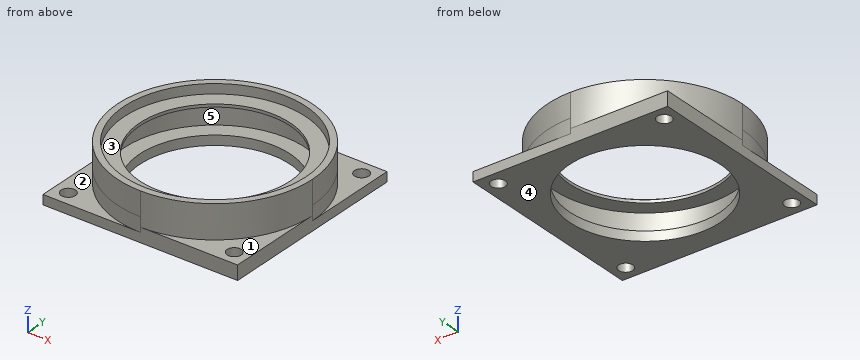
from build123d import *

# Parameters (mm, degrees)
SKETCH2_R               = 20.4
SKETCH2_R_2             = 15.75
SKETCH2_R_3             = 1.5
BOSS_EXTRUDE1_DEPTH     = 5
BOSS_EXTRUDE2_START     = 5
SKETCH2_4_R             = 20.4
SKETCH2_4_R_2           = 15.75
SKETCH2_4_R_3           = 1.5
BOSS_EXTRUDE2_DEPTH     = 6
SKETCH4_R               = 19.05
CUT_EXTRUDE2_DEPTH      = 3
CUT_EXTRUDE3_START      = -6
SKETCH5_R               = 19.05
SKETCH5_R_2             = 15.75
CUT_EXTRUDE3_DEPTH      = 5.4
CUT_EXTRUDE4_START      = -3
CUT_EXTRUDE4_DEPTH      = 3
CUT_EXTRUDE5_START      = -1
SKETCH7_R               = 19.05
CUT_EXTRUDE5_DEPTH      = 1
CUT_EXTRUDE6_DEPTH      = 30.938603842
CUT_EXTRUDE6_DEPTH_BACK = 5


with BuildPart() as part:
    # Sketch2 → Boss-Extrude1 (new body)
    # profile 1 of 5: a face of its own
    with BuildSketch(Plane.XY):
        Circle(SKETCH2_R)
        Circle(SKETCH2_R_2, mode=Mode.SUBTRACT)
    # profile 2 of 5: a face of its own
    with BuildSketch(Plane.XY):
        with BuildLine():
            Line((-20.4, 20.4), (-20.4, -3.8e-08))
            ThreePointArc((-20.4, -3.8e-08), (-14.424978339, 14.424978334), (3.1e-08, 20.4))
            Line((3.1e-08, 20.4), (-20.4, 20.4))
        make_face()
        with Locations((-17.4, 17.4)):
            Circle(SKETCH2_R_3, mode=Mode.SUBTRACT)
    # profile 3 of 5: a face of its own
    with BuildSketch(Plane.XY):
        with BuildLine():
            ThreePointArc((3.1e-08, 20.4), (14.424978347, 14.424978325), (20.4, 0))
            Line((20.4, 0), (20.4, 20.4))
            Line((20.4, 20.4), (3.1e-08, 20.4))
        make_face()
        with Locations((17.4, 17.4)):
            Circle(SKETCH2_R_3, mode=Mode.SUBTRACT)
    # profile 4 of 5: a face of its own
    with BuildSketch(Plane.XY):
        with BuildLine():
            ThreePointArc((20.4, 0), (14.424978335, -14.424978337), (-2e-09, -20.4))
            Line((-2e-09, -20.4), (20.4, -20.4))
            Line((20.4, -20.4), (20.4, 0))
        make_face()
        with Locations((17.4, -17.4)):
            Circle(SKETCH2_R_3, mode=Mode.SUBTRACT)
    # profile 5 of 5: a face of its own
    with BuildSketch(Plane.XY):
        with BuildLine():
            Line((-20.4, -3.8e-08), (-20.4, -20.4))
            Line((-20.4, -20.4), (-2e-09, -20.4))
            ThreePointArc((-2e-09, -20.4), (-14.424978323, -14.424978349), (-20.4, -3.8e-08))
        make_face()
        with Locations((-17.4, -17.4)):
            Circle(SKETCH2_R_3, mode=Mode.SUBTRACT)
    extrude(amount=BOSS_EXTRUDE1_DEPTH)

    # Sketch2<4> → Boss-Extrude2 (add)
    # profile 1 of 3: a face of its own
    with BuildSketch(Plane.XY.offset(BOSS_EXTRUDE2_START)):
        Circle(SKETCH2_4_R)
        Circle(SKETCH2_4_R_2, mode=Mode.SUBTRACT)
    # profile 2 of 3: a face of its own
    with BuildSketch(Plane.XY.offset(BOSS_EXTRUDE2_START)):
        with BuildLine():
            Line((-20.4, 20.4), (-20.4, -3.8e-08))
            ThreePointArc((-20.4, -3.8e-08), (-14.424978339, 14.424978334), (3.1e-08, 20.4))
            Line((3.1e-08, 20.4), (-20.4, 20.4))
        make_face()
        with Locations((-17.4, 17.4)):
            Circle(SKETCH2_4_R_3, mode=Mode.SUBTRACT)
    # profile 3 of 3: a face of its own
    with BuildSketch(Plane.XY.offset(BOSS_EXTRUDE2_START)):
        with BuildLine():
            ThreePointArc((20.4, 0), (14.424978335, -14.424978337), (-2e-09, -20.4))
            Line((-2e-09, -20.4), (20.4, -20.4))
            Line((20.4, -20.4), (20.4, 0))
        make_face()
        with Locations((17.4, -17.4)):
            Circle(SKETCH2_4_R_3, mode=Mode.SUBTRACT)
    extrude(amount=BOSS_EXTRUDE2_DEPTH)

    # Sketch4 → Cut-Extrude2 (cut)
    with BuildSketch(Plane.XY.offset(11)):
        Circle(SKETCH4_R)
    extrude(amount=-CUT_EXTRUDE2_DEPTH, mode=Mode.SUBTRACT)

    # Sketch5 → Cut-Extrude3 (cut)
    with BuildSketch(Plane.XY.offset(8).offset(CUT_EXTRUDE3_START)):
        Circle(SKETCH5_R)
        with Locations(Location((0, 0, 0), (0, 0, 180))):
            Circle(SKETCH5_R_2, mode=Mode.SUBTRACT)
    extrude(amount=CUT_EXTRUDE3_DEPTH, mode=Mode.SUBTRACT)

    # Sketch6 → Cut-Extrude4 (cut)
    with BuildSketch(Plane.XY.offset(5).offset(CUT_EXTRUDE4_START)):
        with BuildLine():
            Line((20.4, 0), (20.4, 20.4))
            Line((20.4, 20.4), (0, 20.4))
            ThreePointArc((0, 20.4), (14.424978336, 14.424978336), (20.4, 0))
        make_face()
        with BuildLine():
            Line((-20.4, 0), (-20.4, -20.4))
            Line((-20.4, -20.4), (0, -20.4))
            ThreePointArc((0, -20.4), (-14.424978336, -14.424978336), (-20.4, 0))
        make_face()
    extrude(amount=CUT_EXTRUDE4_DEPTH, mode=Mode.SUBTRACT)

    # Sketch7 → Cut-Extrude5 (cut)
    with BuildSketch(Plane.XY.offset(11).offset(CUT_EXTRUDE5_START)):
        with BuildLine():
            Line((20.4, -20.4), (20.4, 0))
            ThreePointArc((20.4, 0), (14.424978336, 14.424978336), (0, 20.4))
            Line((0, 20.4), (-20.4, 20.4))
            Line((-20.4, 20.4), (-20.4, 0))
            ThreePointArc((-20.4, 0), (-14.424978336, -14.424978336), (0, -20.4))
            Line((0, -20.4), (20.4, -20.4))
        make_face()
        Circle(SKETCH7_R, mode=Mode.SUBTRACT)
    extrude(amount=CUT_EXTRUDE5_DEPTH, mode=Mode.SUBTRACT)

    # Sketch8 → Cut-Extrude6 (cut, two sides: drawn at the far end of the back side and taken through both)
    with BuildSketch(Plane.XY.offset(8).offset(-CUT_EXTRUDE6_DEPTH_BACK)):
        with BuildLine():
            Line((-20.4, 20.4), (-20.4, 0))
            ThreePointArc((-20.4, 0), (-14.424978336, 14.424978336), (0, 20.4))
            Line((0, 20.4), (-20.4, 20.4))
        make_face()
        with BuildLine():
            ThreePointArc((20.4, 0), (14.424978336, -14.424978336), (0, -20.4))
            Line((0, -20.4), (20.4, -20.4))
            Line((20.4, -20.4), (20.4, 0))
        make_face()
    extrude(amount=CUT_EXTRUDE6_DEPTH + CUT_EXTRUDE6_DEPTH_BACK, mode=Mode.SUBTRACT)


solid = part.part
Can you work these out from the model? Positions are in its coordinate system, mm. Face numbers are marked on the shaded views. A direction names the side the tool comes from. Coordinates: 2 decimals unless noted, no trailing zeros. Write each loop counter-clockwise with the first axis right and the second up, starting at its lowest first coordinate (ties: lowest second). Pieces come first, ordered by that corner, then holes. Notation, with made-up numbers: (68.5, 80) -> (106.5, 80) arc R29 ccw to (106.5, 104) -> close; hole circle Ø11 at (40, 33.5). An arc over 180 degrees is marked (long way). Write item = value, one per line.
(1) On a 3-axis mill with a long thin cutter (end or side, diameter ignored), from which of +Z, -Z, +X, -X, +Y, -Y can I reach the whole of each face in a straight line? I mean the marked faces 1, 2 and 3. Say none if no direction works.
Verdict:
face_1 = +Z, +X, -Y
face_2 = +Z, -X, -Y
face_3 = +Z
(2) Imagine slicing it at C-C (z = 3.5). Please give me the cut outline in (x, y).
Verdict:
outline = circle Ø40.8 at (0, 0); hole circle Ø38.1 at (0, 0)
(3) Thinking about a two-plate mould opening in Y: for the marked faces 4 and 5, which applies, +Y half, -Y half, draft (parallel to the pull), parting line (faces both ways), or undercut?
Verdict:
face_4 = draft
face_5 = undercut
(4) Imagine slicing it at A-A (x = -17.4). Please give me the cut outline in (y, z).
Verdict:
outline = (-20.4, 0) -> (-18.9, 0) -> (-18.9, 2) -> (-20.4, 2) -> close; (-15.9, 0) -> (15.9, 0) -> (15.9, 3) -> (10.65, 3) -> (10.65, 10) -> (7.76, 10) -> (7.76, 8) -> (-7.76, 8) -> (-7.76, 10) -> (-10.65, 10) -> (-10.65, 2) -> (-15.9, 2) -> close; (18.9, 0) -> (20.4, 0) -> (20.4, 3) -> (18.9, 3) -> close; hole (-7.76, 2) -> (7.76, 2) -> (7.76, 7.4) -> (-7.76, 7.4) -> close
(5) For pin 1 (3 mm diameter, centred on x = -15, z = 8.5, fed in from +Y); pin 2 (2 mm diameter, centred on x = -10.5, y = -13.5, fed in from +Z); pin 3 (1 mm diameter, centred on x = -11.5, z = 4.5, fed in from +Y), each with a flat end and sliding along its axis, tell me the tip position at first contact or that it passes through.
Verdict:
pin_1 = 15.29
pin_2 = 8
pin_3 = 17.18
(6) If I drill on probe 1 along X at (y, z) = (17.4, 1.5); probe 2 along X at (y, z) = (0, 7.85), over which ranges is the centre line in solid material (lowest first)?
Verdict:
probe_1 = -20.4 to -18.9, -15.9 to 15.9, 18.9 to 20.4
probe_2 = -20.4 to -15.75, 15.75 to 20.4
(7) Imagine slicing it at D-D (y = 14.5). Please give me the cut outline in (x, z), and give its area (3 significant figures).
Verdict:
outline = (-20.4, 0) -> (-6.15, 0) -> (-6.15, 2) -> (-12.36, 2) -> (-12.36, 7.4) -> (-6.15, 7.4) -> (-6.15, 8) -> (-12.36, 8) -> (-12.36, 10) -> (-14.35, 10) -> (-14.35, 3) -> (-20.4, 3) -> close; (6.15, 0) -> (20.4, 0) -> (20.4, 2) -> (14.35, 2) -> (14.35, 10) -> (12.36, 10) -> (12.36, 8) -> (6.15, 8) -> (6.15, 7.4) -> (12.36, 7.4) -> (12.36, 2) -> (6.15, 2) -> close
area = 102 mm^2
